For this review, take the finished solid that the model builds, in its own axes (mm). Give positions to 0.01 mm unless a question says otherwise; leave off trailing zeros. Write each loop counter-clockwise with the first axis right and the second up, starting at its lowest first coordinate (ties: lowest second). Pieces come first, ordered by that corner, then holes. Notation, with made-up numbers: M 0.5,24 L 24.5,24 A14 ccw 24.5,51 Z; hole C 62.5,20 d6. An arc over 180 degrees is marked long. One line per item, written item: value. Start each with the question number.
Item 1: Mouldability with a two-part tool opening along Y and no side actions: class faces 1 (the face through (31.19, 23.78, 15.62)), 2 (the face through (-4.26, 58.49, 15.62)), 3 (the face through (-45.2, 18.67, 2.96)) as released by +Y, released by -Y, zero draft, split by the parting line, or undercut.
Item 2: Consider section A-A, the plane x = -9. Write out the cut boundary in (y, z).
Item 3: Clearance check with flat-ended pins moving along their axes: pin 1 Ø2 at (y, z) = (14, 8) entering from +X; pin 2 Ø4 at (y, z) = (43, 27) entering from -X; pin 3 Ø2 at (x, z) = (-40.5, 8) entering from +Y; pin 4 Ø5 at (x, y) = (-40.5, -3.5) entering from -Z. State where each tip first meets the part, or that it passes through.
Item 4: Consider section B-B, the plane y = 2.5. Write out the cut boundary in (x, z).
Item 5: To check wall thickness, follow probe 1 along X at (y, z) = (33, 14); probe 2 along Y at (x, z) = (4.5, 5); probe 3 along X at (y, z) = (41.5, 19.5). State the ranges of each line that lie inside material, in increasing order.
```python
from build123d import *

# Parameters (mm, degrees)
SKETCH1_W           = 73.7
SKETCH1_H           = 74.3
BOSS_EXTRUDE1_DEPTH = 31.69
BOSS_EXTRUDE1_TAPER = 7
SKETCH2_R           = 1.5
BOSS_EXTRUDE2_DEPTH = 10
SKETCH3_R           = 1.5
BOSS_EXTRUDE3_DEPTH = 10
SKETCH4_R           = 1.5
BOSS_EXTRUDE4_DEPTH = 10
SKETCH5_R           = 1.5
BOSS_EXTRUDE5_DEPTH = 10


with BuildPart() as part:
    # Sketch1 → Boss-Extrude1 (new body)
    with BuildSketch(Plane.XY):
        with Locations((-3.742578125, 23.259277344)):
            Rectangle(SKETCH1_W, SKETCH1_H)
    extrude(amount=BOSS_EXTRUDE1_DEPTH, taper=BOSS_EXTRUDE1_TAPER)

    # Sketch2 → Boss-Extrude2 (add)
    with BuildSketch(Plane(origin=(-39.989691599, 0, 4.910116724), x_dir=(0.1218693434051475, 0, 0.992546151641322), z_dir=(-0.992546151641322, 0, 0.1218693434051475))):
        with Locations((-2.003690491, 35.125279491)):
            Circle(SKETCH2_R)
    extrude(amount=BOSS_EXTRUDE2_DEPTH)

    # Sketch3 → Boss-Extrude3 (add)
    with BuildSketch(Plane(origin=(-39.989691599, 0, 4.910116724), x_dir=(0.1218693434051475, 0, 0.992546151641322), z_dir=(-0.992546151641322, 0, 0.1218693434051475))):
        with Locations((-2.079096661, 29.570839743)):
            Circle(SKETCH3_R)
    extrude(amount=BOSS_EXTRUDE3_DEPTH)

    # Sketch4 → Boss-Extrude4 (add)
    with BuildSketch(Plane(origin=(-39.989691599, 0, 4.910116724), x_dir=(0.1218693434051475, 0, 0.992546151641322), z_dir=(-0.992546151641322, 0, 0.1218693434051475))):
        with Locations((-2.088291419, 24.676586011)):
            Circle(SKETCH4_R)
    extrude(amount=BOSS_EXTRUDE4_DEPTH)

    # Sketch5 → Boss-Extrude5 (add)
    with BuildSketch(Plane(origin=(-39.989691599, 0, 4.910116724), x_dir=(0.1218693434051475, 0, 0.992546151641322), z_dir=(-0.992546151641322, 0, 0.1218693434051475))):
        with Locations((-2.246014271, 20.134764101)):
            Circle(SKETCH5_R)
    extrude(amount=BOSS_EXTRUDE5_DEPTH)


solid = part.part
```
Model answer:
1. face 1: zero draft
1. face 2: released by +Y
1. face 3: undercut
2. outline: M -13.89,0 L 60.41,0 L 56.52,31.69 L -10,31.69 Z
3. pin 1: stops at x = 32.25
3. pin 2: stops at x = -37.52
3. pin 3: stops at y = 59.5
3. pin 4: stops at z = 0
4. outline: M -40.59,0 L 33.11,0 L 29.22,31.69 L -36.7,31.69 Z
5. probe 1: x = -38.87 to 31.39
5. probe 2: y = -13.28 to 59.8
5. probe 3: x = -38.2 to 30.71
